from build123d import *

# Parameters (mm, degrees)
SZKIC4_R                    = 2.25
DODANIE_WYCI_GNI_CIE1_DEPTH = 1.875


with BuildPart() as part:
    # Szkic1 → Obr_t1 (revolve)
    with BuildSketch(Plane.XY, mode=Mode.PRIVATE) as obr_t1_sk:
        Polygon((0, 0), (0, 4), (0.3, 4), (2.3, 2), (2.3, 0), align=None)
    revolve(obr_t1_sk.sketch.rotate(Axis((2.3, 0, 0), (-1, 0, 0)), 270), axis=Axis((2.3, 0, 0), (-1, 0, 0)))

    # Szkic2 → Obr_t2 (revolve)
    with BuildSketch(Plane.XY, mode=Mode.PRIVATE) as obr_t2_sk:
        Polygon((2.3, 0), (2.3, 2), (7.5705, 2), (8, 1.5705), (8, 0), align=None)
    revolve(obr_t2_sk.sketch.rotate(Axis((8, 0, 0), (-1, 0, 0)), 270), axis=Axis((8, 0, 0), (-1, 0, 0)))

    # Szkic3 → Wyci_cie-obr_t1 (revolve, cut)
    with BuildSketch(Plane.XY, mode=Mode.PRIVATE) as wyci_cie_obr_t1_sk:
        Polygon((0, 0), (0, 1.95), (1.5, 1.95), (2.625833025, 0), align=None)
    revolve(wyci_cie_obr_t1_sk.sketch.rotate(Axis((2.625833025, 0, 0), (-1, 0, 0)), 270), axis=Axis((2.625833025, 0, 0), (-1, 0, 0)), mode=Mode.SUBTRACT)

    # Szkic4 → Dodanie-wyci_gni_cie1 (add)
    with BuildSketch(Plane(origin=(0, 0, 0), x_dir=(0, 0, -1), z_dir=(1, 0, 0))):
        Circle(SZKIC4_R)
        Polygon((-1.25, 0.721687836), (-1.25, -0.721687836), (0, -1.443375673), (1.25, -0.721687836), (1.25, 0.721687836), (0, 1.443375673), align=None, mode=Mode.SUBTRACT)
    extrude(amount=DODANIE_WYCI_GNI_CIE1_DEPTH)


solid = part.part
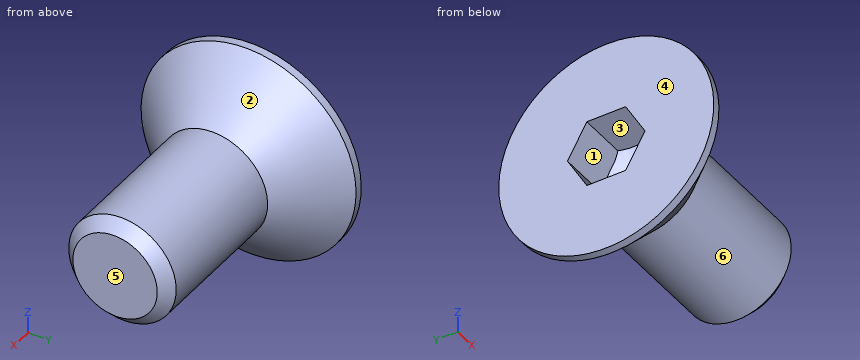
The listing builds one solid part. Answer for the finished solid, in the listing's coordinates (mm). Face numbers are marked on the shaded views. A direction names the side the tool comes from. Coordinates: 2 decimals unless noted, no trailing zeros. Loops run counter-clockwise (first coordinate to the right, second up) from the corner with the lowest first, then second, coordinate; pieces in that order, holes last.
1) Flat-ended cylindrical pins translate along their axes: pin 1 Ø1.5 at (x, z) = (6.5, 3) entering from -Y; pin 2 Ø1.2 at (x, y) = (1, -0.5) entering from -Z; pin 3 Ø3 at (x, z) = (6.5, -3) entering from +Y; pin 4 Ø3 at (x, z) = (3.5, -2) entering from -Y. Find the tip coordinate at first contact, or state that the pin passes through.
2) Find the intervals of material crossed by L1, parallel to Y at x = 2, z = 0.5 (3 decimals); L2, parallel to X at y = -0.25, z = -0.5; L3, parallel to Z at x = 1.5, y = -2.5, in increasing order.
3) A tool of negligible diameter and unlimited length cuts with its end or side. For the marked faces 5 and 6, from which of +Z, -Z, +X, -X, +Y, -Y can it reach the whole face along a straight path? Write none if from no direction.
4) Determine the mould class of the marked faces 1, 2, 3 and 4 for opening direction Z: pulls with the +Z half, pulls with the -Z half, needs draft (parallel to the pull), parting line crosses it, or undercut.
5) Find section A-A on x = 5.75. Write down the section's boundary in (y, z), then the cut area to 3 significant figures.
Values:
1. pin 1: passes through
1. pin 2: stops at z = -3.87
1. pin 3: stops at y = 1.32
1. pin 4: stops at y = -1.94
2. L1: y = -2.245 to -0.962, 0.962 to 2.245
2. L2: x = 2.3 to 8
2. L3: z = -1.26 to 1.26
3. face 5: +Z, -Z, +X, +Y, -Y
3. face 6: +X
4. face 1: undercut
4. face 2: parting line crosses it
4. face 3: undercut
4. face 4: needs draft
5. outline: circle Ø4 at (0, 0)
5. area: 12.6 mm2
